Input: part model. Units: mm. Frame: model coordinates. Face numbers are marked on the shaded views. A direction names the side the tool comes from. Give positions to 0.01 mm unless a question says otherwise; leave off trailing zeros. Loops run counter-clockwise (first coordinate to the right, second up) from the corner with the lowest first, then second, coordinate; pieces in that order, holes last. Notation, with made-up numbers: M 32.25,-10.75 L 80.25,-10.75 A25 ccw 80.25,22.25 Z; hole C 30,63.5 d6. An arc over 180 degrees is marked long. One line per item, written item: value. Start each with the question number.
(1) Ray query, line 1 along Y through (x, z) = (-0.25, 130); line 2 along Y through (x, z) = (0, 92) (3 decimals); line 3 along Z through (x, y) = (6, -2.25). Return the intervals inside material, ascending. Write a range as from..to.
(2) Section A-A on z = -8. Output: boundary loops of the cut face in (x, y).
(3) Pin query (flat end, axial travel): P1, Ø1, axis at x = -4.5, y = -5, coming from the +Z side; P2, Ø6, axis at y = 4, z = 116, coming from the +X side; P3, Ø1.3, axis at x = 1, y = 0.5, coming from the +Z side. Return the tip coordinate at first contact, or that it passes through.
(4) Access query for the marked faces 1 and 2. Directions: +Z, -Z, +X, -X, +Y, -Y. A direction counts if a zero-diameter tool reaches every point of the face in a straight line with its end or side. Return the directions, or none.
(5) Section B-B on x = 0.25. Output: boundary loops of the cut face in (y, z), plus the area to 3 significant figures.
(6) Section C-C on z = 57. Output: boundary loops of the cut face in (x, y) (3 decimals).
Autodesk Inventor part; units mm, degrees
ref_plane "YZ Plane" through (0, 0, 0) normal (1, 0, 0) x (0, 1, 0)
ref_plane "XZ Plane" through (0, 0, 0) normal (0, 1, 0) x (-1, 0, 0)
ref_plane "XY Plane" through (0, 0, 0) normal (0, 0, 1) x (1, 0, 0)
sketch "Sketch1" plane through (0, 0, 0) normal (0, 0, 1) x (1, 0, 0)
  circle A0 centre (0, 0) radius 7.875
  dimension "d0" = 15.75
extrude "Extrusion1" add sketch "Sketch1" along normal blind 126
sketch "Sketch2" plane through (0, 0, 126) normal (0, 0, 1) x (1, 0, 0)
  circle A0 centre (0, 0) radius 5.5
  dimension "d3" = 11
extrude "Extrusion2" add sketch "Sketch2" along normal blind 10
sketch "Sketch3" plane through (0, 0, 0) normal (0, 0, -1) x (-1, 0, 0)
  circle A0 centre (0, 0) radius 5.5
  dimension "d6" = 11
extrude "Extrusion3" add sketch "Sketch3" along normal blind 14
sketch "Sketch4" plane through (0, 0, -14) normal (0, 0, -1) x (-1, 0, 0)
  line L0 (4, 13.3221) -> (11.8644, 13.3221)
  line L1 (11.8644, 13.3221) -> (11.8644, -10.8813)
  line L2 (11.8644, -10.8813) -> (4, -10.8813)
  line L3 (4, -10.8813) -> (4, 13.3221)
  line L4 (-11.0508, 13.3221) -> (-4, 13.3221)
  line L5 (-4, 13.3221) -> (-4, -10.8813)
  line L6 (-4, -10.8813) -> (-11.0508, -10.8813)
  line L7 (-11.0508, -10.8813) -> (-11.0508, 13.3221)
  point P0 (0, 0)
  dimension "d9" = 8
  dimension "d10" = 4
extrude "Extrusion4" cut sketch "Sketch4" against normal up to surface (14 mm away)
sketch "Sketch5" plane through (4, -3.7749, -14) normal (1, 0, 0) x (0, 0, -1)
  circle A0 centre (-6, 3.7748) radius 2
  line L0 (0, 7.5498) -> (0, 0)
  line L1 (-14, 7.5498) -> (0, 7.5498)
  point P0 (-14, 3.7749)
  dimension "d13" = 4
  dimension "d14" = 6
  dimension "d15" = 3.775
extrude "Extrusion5" cut sketch "Sketch5" against normal up to next
sketch "Sketch7" plane through (0, 0, 136) normal (0, 0, 1) x (1, 0, 0)
  circle A0 centre (0, 0) radius 2.25
  dimension "d21" = 4.5
extrude "Extrusion7" cut sketch "Sketch7" against normal blind 140
properties part number "Small_piston" material "Aluminum 6061-AHC"
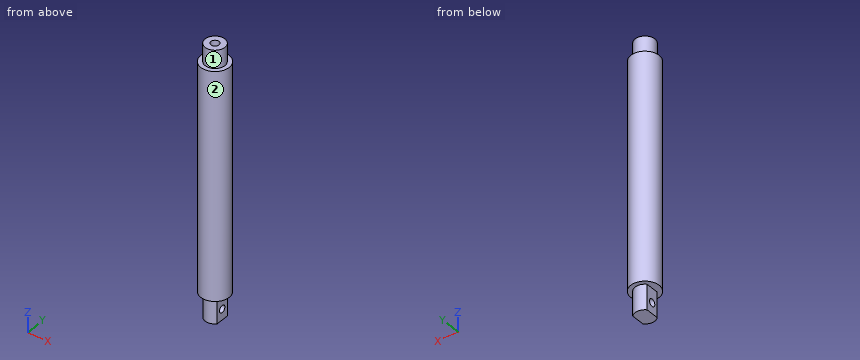
Output values:
1. line 1: y = -5.49..-2.24, 2.24..5.49
1. line 2: y = -7.875..-2.25, 2.25..7.875
1. line 3: z = 0..126
2. outline: M -4,-3.77 A5.5 ccw 4,-3.77 L 4,-2 L -4,-2 Z; M -4,2 L 4,2 L 4,3.77 A5.5 ccw -4,3.77 Z
3. P1: stops at z = 126
3. P2: stops at x = 7.81
3. P3: stops at z = -4
4. face 1: +Z
4. face 2: +Z, -Z
5. outline: M -7.87,0 L -5.49,0 L -5.49,-14 L 5.49,-14 L 5.49,0 L 7.87,0 L 7.87,126 L 5.49,126 L 5.49,136 L 2.24,136 L 2.24,-4 L -2.24,-4 L -2.24,136 L -5.49,136 L -5.49,126 L -7.87,126 Z; hole C 0,-8 d4
5. area: 1,610 mm²
6. outline: C 0,0 d15.75; hole C 0,0 d4.5
